Could you check a few things on this model? Use its own coordinates, in mm. A direction names the side the tool comes from. Give positions to 0.01 mm unless a question says otherwise; leave off trailing zeros. Write each loop counter-clockwise with the first axis right and the second up, starting at its lowest first coordinate (ties: lowest second). Pieces come first, ordered by that corner, then holes. Notation, with made-up numbers: M -33.75,-3.5 L -8.75,-3.5 A19 cw -8.75,24.5 Z; hole C 29.25,-5.75 d2. An arc over 180 degrees is marked long. One line per item, written item: value.
```python
from build123d import *

# Parameters (mm, degrees)
SKETCH1_R           = 1.5494
SKETCH1_R_2         = 1.778
BOSS_EXTRUDE1_DEPTH = 3.175
FILLET2_R           = 2.54
FILLET3_R           = 2.54


with BuildPart() as part:
    # Sketch1 → Boss-Extrude1 (new body)
    with BuildSketch(Plane.XY):
        Polygon((0.381, 116.2304), (105.391042757, 116.2304), (105.391042757, 101.985486737), (151.460414906, 101.985486737), (151.460414906, 116.2304), (175.133, 116.2304), (175.133, 0.4064), (0.381, 0.4064), align=None)
        with Locations((6.4516, 109.3724)):
            Circle(SKETCH1_R, mode=Mode.SUBTRACT)
        with Locations((169.4688, 104.6734)):
            Circle(SKETCH1_R, mode=Mode.SUBTRACT)
        with Locations((169.4688, 14.0208)):
            Circle(SKETCH1_R, mode=Mode.SUBTRACT)
        with Locations((6.4516, 25.0952)):
            Circle(SKETCH1_R, mode=Mode.SUBTRACT)
        with Locations((15.748, 112.649)):
            Circle(SKETCH1_R_2, mode=Mode.SUBTRACT)
        with Locations((159.004, 112.649)):
            Circle(SKETCH1_R_2, mode=Mode.SUBTRACT)
        with Locations((15.748, 9.271)):
            Circle(SKETCH1_R_2, mode=Mode.SUBTRACT)
        with Locations(Location((159.004, 9.271, 0), (0, 0, 180))):
            Circle(SKETCH1_R_2, mode=Mode.SUBTRACT)
        with BuildLine():
            Line((44.96589092, 70.321337511), (44.96589092, 69.559337511))
            ThreePointArc((44.96589092, 69.559337511), (45.412260185, 68.481706777), (46.48989092, 68.035337511))
            Line((46.48989092, 68.035337511), (128.26210908, 68.035337511))
            ThreePointArc((128.26210908, 68.035337511), (129.339739815, 68.481706777), (129.78610908, 69.559337511))
            Line((129.78610908, 69.559337511), (129.78610908, 70.321337511))
            ThreePointArc((129.78610908, 70.321337511), (129.339739815, 71.398968246), (128.26210908, 71.845337511))
            Line((128.26210908, 71.845337511), (46.48989092, 71.845337511))
            ThreePointArc((46.48989092, 71.845337511), (45.412260185, 71.398968246), (44.96589092, 70.321337511))
        make_face(mode=Mode.SUBTRACT)
        with BuildLine():
            Line((46.48989092, 79.465337511), (128.26210908, 79.465337511))
            ThreePointArc((128.26210908, 79.465337511), (129.339739815, 79.018968246), (129.78610908, 77.941337511))
            Line((129.78610908, 77.941337511), (129.78610908, 77.179337511))
            ThreePointArc((129.78610908, 77.179337511), (129.339739815, 76.101706777), (128.26210908, 75.655337511))
            Line((128.26210908, 75.655337511), (46.48989092, 75.655337511))
            ThreePointArc((46.48989092, 75.655337511), (45.412260185, 76.101706777), (44.96589092, 77.179337511))
            Line((44.96589092, 77.179337511), (44.96589092, 77.941337511))
            ThreePointArc((44.96589092, 77.941337511), (45.412260185, 79.018968246), (46.48989092, 79.465337511))
        make_face(mode=Mode.SUBTRACT)
        with BuildLine():
            Line((44.96589092, 62.701337511), (44.96589092, 61.939337511))
            ThreePointArc((44.96589092, 61.939337511), (45.412260185, 60.861706777), (46.48989092, 60.415337511))
            Line((46.48989092, 60.415337511), (128.26210908, 60.415337511))
            ThreePointArc((128.26210908, 60.415337511), (129.339739815, 60.861706777), (129.78610908, 61.939337511))
            Line((129.78610908, 61.939337511), (129.78610908, 62.701337511))
            ThreePointArc((129.78610908, 62.701337511), (129.339739815, 63.778968246), (128.26210908, 64.225337511))
            Line((128.26210908, 64.225337511), (46.48989092, 64.225337511))
            ThreePointArc((46.48989092, 64.225337511), (45.412260185, 63.778968246), (44.96589092, 62.701337511))
        make_face(mode=Mode.SUBTRACT)
        with BuildLine():
            Line((44.96589092, 55.081337511), (44.96589092, 54.319337511))
            ThreePointArc((44.96589092, 54.319337511), (45.412260185, 53.241706777), (46.48989092, 52.795337511))
            Line((46.48989092, 52.795337511), (128.26210908, 52.795337511))
            ThreePointArc((128.26210908, 52.795337511), (129.339739815, 53.241706777), (129.78610908, 54.319337511))
            Line((129.78610908, 54.319337511), (129.78610908, 55.081337511))
            ThreePointArc((129.78610908, 55.081337511), (129.339739815, 56.158968246), (128.26210908, 56.605337511))
            Line((128.26210908, 56.605337511), (46.48989092, 56.605337511))
            ThreePointArc((46.48989092, 56.605337511), (45.412260185, 56.158968246), (44.96589092, 55.081337511))
        make_face(mode=Mode.SUBTRACT)
        with BuildLine():
            Line((44.96589092, 47.461337511), (44.96589092, 46.699337511))
            ThreePointArc((44.96589092, 46.699337511), (45.412260185, 45.621706777), (46.48989092, 45.175337511))
            Line((46.48989092, 45.175337511), (128.26210908, 45.175337511))
            ThreePointArc((128.26210908, 45.175337511), (129.339739815, 45.621706777), (129.78610908, 46.699337511))
            Line((129.78610908, 46.699337511), (129.78610908, 47.461337511))
            ThreePointArc((129.78610908, 47.461337511), (129.339739815, 48.538968246), (128.26210908, 48.985337511))
            Line((128.26210908, 48.985337511), (46.48989092, 48.985337511))
            ThreePointArc((46.48989092, 48.985337511), (45.412260185, 48.538968246), (44.96589092, 47.461337511))
        make_face(mode=Mode.SUBTRACT)
        with BuildLine():
            Line((44.96589092, 39.841337511), (44.96589092, 39.079337511))
            ThreePointArc((44.96589092, 39.079337511), (45.412260185, 38.001706777), (46.48989092, 37.555337511))
            Line((46.48989092, 37.555337511), (128.26210908, 37.555337511))
            ThreePointArc((128.26210908, 37.555337511), (129.339739815, 38.001706777), (129.78610908, 39.079337511))
            Line((129.78610908, 39.079337511), (129.78610908, 39.841337511))
            ThreePointArc((129.78610908, 39.841337511), (129.339739815, 40.918968246), (128.26210908, 41.365337511))
            Line((128.26210908, 41.365337511), (46.48989092, 41.365337511))
            ThreePointArc((46.48989092, 41.365337511), (45.412260185, 40.918968246), (44.96589092, 39.841337511))
        make_face(mode=Mode.SUBTRACT)
    extrude(amount=BOSS_EXTRUDE1_DEPTH)

    # Fillet2
    fillet2_edges = [part.edges().sort_by_distance(p)[0] for p in [
        (105.391042757, 116.2304, 1.5875),
        (105.391042757, 101.985486737, 1.5875),
        (151.460414906, 101.985486737, 1.5875),
        (151.460414906, 116.2304, 1.5875),
    ]]
    fillet(fillet2_edges, radius=FILLET2_R)

    # Fillet3
    fillet3_edges = [part.edges().sort_by_distance(p)[0] for p in [
        (0.381, 116.2304, 1.5875),
        (175.133, 116.2304, 1.5875),
        (175.133, 0.4064, 1.5875),
        (0.381, 0.4064, 1.5875),
    ]]
    fillet(fillet3_edges, radius=FILLET3_R)


solid = part.part
```
1) If we section it at B-B, the plane x = 122: Write out the boundary of the cut face in (y, z) (3 decimals).
Outcome:
outline: M 0.406,0 L 37.555,0 L 37.555,3.175 L 0.406,3.175 Z; M 41.365,0 L 45.175,0 L 45.175,3.175 L 41.365,3.175 Z; M 48.985,0 L 52.795,0 L 52.795,3.175 L 48.985,3.175 Z; M 56.605,0 L 60.415,0 L 60.415,3.175 L 56.605,3.175 Z; M 64.225,0 L 68.035,0 L 68.035,3.175 L 64.225,3.175 Z; M 71.845,0 L 75.655,0 L 75.655,3.175 L 71.845,3.175 Z; M 79.465,0 L 101.985,0 L 101.985,3.175 L 79.465,3.175 Z
2) We'd pull the mould along X, two halves only. Please class faces 1 (the face through (151.46, 109, 2)), 2 (the face through (89, 59, 0)), 3 (the face through (175.133, 59, 2)): pulls with the +X half, pulls with the -X half, needs draft (parallel to the pull), parting line crosses it, or undercut.
Outcome:
face 1: undercut
face 2: needs draft
face 3: pulls with the +X half
3) On a 3-axis mill with a long thin cutter (end or side, diameter ignored), from which of +Z, -Z, +X, -X, +Y, -Y can I reach the whole of each face in a straight line? I mean faces 4 (the face through (128, 101.985, 2)), 5 (the face through (163, 116.23, 2)), 6 (the face through (87, 60.415, 2)). Say none if no direction works.
Outcome:
face 4: +Z, -Z, +Y
face 5: +Z, -Z, +X, -X, +Y
face 6: +Z, -Z
4) Please list where these lines run through material, in increasing order: L1, parallel to X at y = 70, z = 2.2; L2, parallel to Y at x = 130.5, z = 2.65; L3, parallel to X at y = 61.5, z = 1.15. Write a range as from..to.
Outcome:
L1: x = 0.38..44.97, 129.79..175.13
L2: y = 0.41..101.99
L3: x = 0.38..45.03, 129.72..175.13
5) If we section it at C-C, the plane z = 1.7: Give the number of separate pieces and of enclosed holes in the cut face, then the cut area to 3 significant figures.
Outcome:
separate pieces: 1
enclosed holes: 14
area: 17,600 mm^2
6) If we section it at A-A, the plane x = 82.5: Write out the boundary of the cut face in (y, z) (3 decimals), then the cut area to 3 significant figures.
Outcome:
outline: M 0.406,0 L 37.555,0 L 37.555,3.175 L 0.406,3.175 Z; M 41.365,0 L 45.175,0 L 45.175,3.175 L 41.365,3.175 Z; M 48.985,0 L 52.795,0 L 52.795,3.175 L 48.985,3.175 Z; M 56.605,0 L 60.415,0 L 60.415,3.175 L 56.605,3.175 Z; M 64.225,0 L 68.035,0 L 68.035,3.175 L 64.225,3.175 Z; M 71.845,0 L 75.655,0 L 75.655,3.175 L 71.845,3.175 Z; M 79.465,0 L 116.23,0 L 116.23,3.175 L 79.465,3.175 Z
area: 295 mm^2
7) I'm going to push a flat-ended pin straight in: pin 1 (1.6 mm diameter, centred on x = 126.5, z = 2.5, fed in from +Y). Where does the tip first touch, or does it pass through?
Outcome:
pin 1: stops at y = 101.99
